Geometry: final body of the model. Coordinates: model frame, mm. A direction names the side the tool comes from. Coordinates: 2 decimals unless noted, no trailing zeros. Order: outer loops, then holes, each group sorted by start corner. A loop starts at its lowest first (then second) coordinate and runs counter-clockwise, first axis right, second up. Notation, with made-up numbers: M 21,-21 L 68,-21 A21 cw 68,4 Z; hole C 3.5,22.25 d2. An arc over 180 degrees is marked long. One line per question, with ' | ' between items.
from build123d import *

# Parameters (mm, degrees)
BOSS_EXTRUDE1_DEPTH  = 60
M6_CLEARANCE_HOLE1_D = 6.6


with BuildPart() as part:
    # Sketch1 → Boss-Extrude1 (new body)
    with BuildSketch(Plane.XY):
        with BuildLine():
            Line((971.299999999, 2378.548566852), (895.5, 2378.548566852))
            Line((895.5, 2378.548566852), (895.5, 2258.548566852))
            Line((895.5, 2258.548566852), (895.5, 2138.548566852))
            Line((895.5, 2138.548566852), (971.299999999, 2138.548566852))
            Line((971.299999999, 2138.548566852), (971.299999999, 2181.347801943))
            ThreePointArc((971.299999999, 2181.347801943), (984.737192979, 2219.081914402), (1018.999999999, 2239.829961379))
            Line((1018.999999999, 2239.829961379), (1018.999999999, 2277.267172325))
            ThreePointArc((1018.999999999, 2277.267172325), (984.737192979, 2298.015219302), (971.299999999, 2335.749331762))
            Line((971.299999999, 2335.749331762), (971.299999999, 2378.548566852))
        make_face()
    extrude(amount=BOSS_EXTRUDE1_DEPTH)

    # M6 Clearance Hole1 (through all)
    with Locations(Plane.XY.offset(60)):
        with Locations((901.5, 2145.048566852), (958.5, 2145.048566852), (958.5, 2190.048566852), (901.5, 2190.048566852), (901.5, 2372.048566852), (901.5, 2327.048566852), (958.5, 2327.048566852), (958.5, 2372.048566852), (1013.999999999, 2247.548566852), (1013.999999999, 2269.548566852), (975.999999999, 2247.548566852), (975.999999999, 2269.548566852)):
            Hole(M6_CLEARANCE_HOLE1_D / 2)


solid = part.part
1. Section C-C, the plane z = 11. Give the number of separate pieces and of enclosed holes in the cut face, and give its area (3 significant figures).
Response values:
separate pieces: 1 | enclosed holes: 12 | area: 21,000 mm^2
2. Access query for faces 5 (the face through (971.3, 2357, 30)), 6 (the face through (902.22, 2141.83, 29.58)), 7 (the face through (971.3, 2160, 30)). Directions: +Z, -Z, +X, -X, +Y, -Y. A direction counts if a zero-diameter tool reaches every point of the face in a straight line with its end or side. Return the directions, or none.
Response values:
face 5: +Z, -Z, +X, +Y | face 6: +Z, -Z | face 7: +Z, -Z, +X, -Y
3. Section A-A, the plane x = 958.5. Output: boundary loops of the cut face in (y, z).
Response values:
outline: M 2138.55,0 L 2141.75,0 L 2141.75,60 L 2138.55,60 Z; M 2148.35,0 L 2186.75,0 L 2186.75,60 L 2148.35,60 Z; M 2193.35,0 L 2323.75,0 L 2323.75,60 L 2193.35,60 Z; M 2330.35,0 L 2368.75,0 L 2368.75,60 L 2330.35,60 Z; M 2375.35,0 L 2378.55,0 L 2378.55,60 L 2375.35,60 Z
4. Pin query (flat end, axial travel): P1, Ø13, axis at y = 2353, z = 15, coming from the +X side; P2, Ø12, axis at x = 996, z = 41.5, coming from the -Y side; P3, Ø1.5, axis at x = 977, z = 33.5, coming from the -Y side. Return the tip coordinate at first contact, or that it passes through.
Response values:
P1: stops at x = 971.3 | P2: stops at y = 2224.74 | P3: stops at y = 2205.15
5. Material intervals for line 1 (Y direction, x = 901.5, z = 17.5); line 2 (X direction, y = 2269, z = 23); line 3 (X direction, y = 2325, z = 26), sorted ascending. Write a range as [from, to].
Response values:
line 1: y = [2138.55, 2141.75], [2148.35, 2186.75], [2193.35, 2323.75], [2330.35, 2368.75], [2375.35, 2378.55] | line 2: x = [895.5, 972.75], [979.25, 1010.75], [1017.25, 1019] | line 3: x = [895.5, 898.91], [904.09, 955.91], [961.09, 972.28]
6. Section D-D, the plane y = 2285. Output: boundary loops of the cut face in (x, z), and give its area (3 significant figures).
Response values:
outline: M 895.5,0 L 999.56,0 L 999.56,60 L 895.5,60 Z | area: 6,240 mm^2
7. Draft query along X for faces 1 (the face through (985.101, 2297.574, 29.58)), 2 (the face through (943, 2260, 60)), 3 (the face through (976.72, 2266.33, 29.58)), 4 (the face through (959.22, 2141.83, 29.58)). Return one class per face: pulls with the +X half, pulls with the -X half, needs draft (parallel to the pull), parting line crosses it, or undercut.
Response values:
face 1: pulls with the +X half | face 2: needs draft | face 3: undercut | face 4: undercut
8. Section B-B, the plane x = 1014. Output: boundary loops of the cut face in (y, z).
Response values:
outline: M 2238.58,0 L 2244.25,0 L 2244.25,60 L 2238.58,60 Z; M 2250.85,0 L 2266.25,0 L 2266.25,60 L 2250.85,60 Z; M 2272.85,0 L 2278.52,0 L 2278.52,60 L 2272.85,60 Z
